Work out the finished part from the listing and answer in its coordinate system (mm). Face numbers are marked on the shaded views. A direction names the side the tool comes from. Round coordinates to 2 decimals unless told otherwise and drop trailing zeros. Order: outer loops, then holes, each group sorted by start corner. A loop starts at its lowest first (then second) coordinate and runs counter-clockwise, first axis right, second up. Notation, with made-up numbers: (-31, -16.75) - (18, -16.75) arc R21 ccw to (18, 5.25) - close; hole circle Ø7 at (86.5, -6.5). An arc over 180 degrees is marked (long way). Answer in a Markdown table with one row per item.
from build123d import *

# Parameters (mm, degrees)
SZKIC1_R                    = 15
DODANIE_WYCI_GNI_CIE1_DEPTH = 53
SFAZOWANIE1_SIZE            = 1
WYTNIJ_WYCI_GNI_CIE1_DEPTH  = 35
SZKIC3_R                    = 30
DODANIE_WYCI_GNI_CIE2_DEPTH = 10
SZKIC4_R                    = 2.5
WYTNIJ_WYCI_GNI_CIE2_DEPTH  = 61.406953242
SZYK_KO_OWY1_COUNT          = 6


with BuildPart() as part:
    # Szkic1 → Dodanie-wyciągnięcie1 (new body)
    with BuildSketch(Plane.XY):
        Circle(SZKIC1_R)
    extrude(amount=DODANIE_WYCI_GNI_CIE1_DEPTH)

    # Sfazowanie1
    sfazowanie1_edges = [part.edges().sort_by_distance(p)[0] for p in [
        (-15, 0, 0),
    ]]
    chamfer(sfazowanie1_edges, length=SFAZOWANIE1_SIZE)

    # Szkic2 → Wytnij-wyciągnięcie1 (cut)
    with BuildSketch(Plane(origin=(0, 0, 4), x_dir=(-1, 0, 0), z_dir=(0, 0, -1))):
        with BuildLine():
            Line((-2.39, 14.808372632), (-2.39, 12.418372632))
            Line((-2.39, 12.418372632), (2.39, 12.418372632))
            Line((2.39, 12.418372632), (2.39, 14.808372632))
            ThreePointArc((2.39, 14.808372632), (0, 15), (-2.39, 14.808372632))
        make_face()
    extrude(amount=-WYTNIJ_WYCI_GNI_CIE1_DEPTH, mode=Mode.SUBTRACT)

    # Szkic3 → Dodanie-wyciągnięcie2 (add)
    with BuildSketch(Plane.XY.offset(53)):
        Circle(SZKIC3_R)
    extrude(amount=-DODANIE_WYCI_GNI_CIE2_DEPTH)

    # Szkic4 → Wytnij-wyciągnięcie2 (cut, through all)
    with BuildSketch(Plane(origin=(0, 0, 43), x_dir=(-1, 0, 0), z_dir=(0, 0, -1))):
        with Locations((-25, 0)):
            Circle(SZKIC4_R)
    wytnij_wyci_gni_cie2 = extrude(amount=-WYTNIJ_WYCI_GNI_CIE2_DEPTH, mode=Mode.SUBTRACT)

    # Szyk kołowy1: Wytnij-wyciągnięcie2 ×6 about axis
    szyk_ko_owy1_axis = Axis((0, 0, 0), (0, 0, 1))
    for i in range(1, SZYK_KO_OWY1_COUNT):
        add(wytnij_wyci_gni_cie2.rotate(szyk_ko_owy1_axis, i * 360 / SZYK_KO_OWY1_COUNT), mode=Mode.SUBTRACT)


solid = part.part
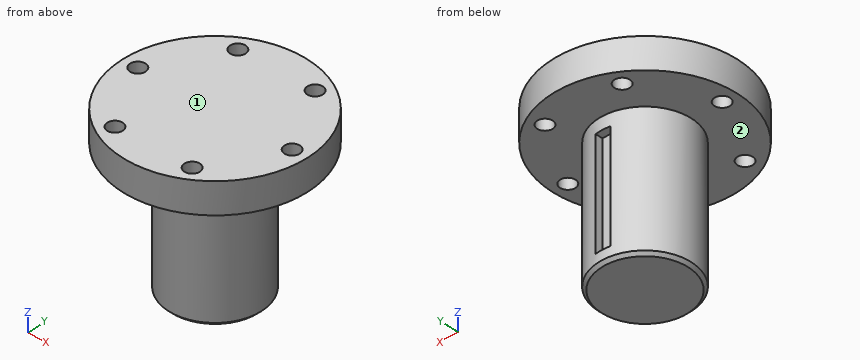
1) Find the intervals of material crossed by probe 1 along Y at (x, z) = (-11, 43.5); probe 2 along Y at (x, z) = (12, 49); probe 3 along Z at (x, y) = (20.5, 8), in increasing order. Write a range as from..to.
Filled in:
| item | result |
|---|---|
| probe 1 | y = -27.91..-23.65, -19.65..19.65, 23.65..27.91 |
| probe 2 | y = -27.5..-24.1, -19.2..19.2, 24.1..27.5 |
| probe 3 | z = 43..53 |
2) Find section B-B, the plane x = 0. Give the vertices of the cut face in (y, z), then the cut area to 3 significant figures.
Filled in:
| item | result |
|---|---|
| outline | (-30, 43) - (-15, 43) - (-15, 1) - (-14, 0) - (14, 0) - (15, 1) - (15, 4) - (12.42, 4) - (12.42, 39) - (15, 39) - (15, 43) - (30, 43) - (30, 53) - (-30, 53) - close |
| area | 1,800 mm^2 |
3) Which of the six approach directions +Z, -Z, +X, -X, +Y, -Y give full straight-line access (tool end or side, diameter ignored) to the marked faces 1 and 2?
Filled in:
| item | result |
|---|---|
| face 1 | +Z, +X, -X, +Y, -Y |
| face 2 | -Z |
4) Find section A-A, the plane y = 0. Give the vertices of the cut face in (x, z), then the cut area to 3 significant figures.
Filled in:
| item | result |
|---|---|
| outline | (-30, 43) - (-27.5, 43) - (-27.5, 53) - (-30, 53) - close; (-22.5, 43) - (-15, 43) - (-15, 1) - (-14, 0) - (14, 0) - (15, 1) - (15, 43) - (22.5, 43) - (22.5, 53) - (-22.5, 53) - close; (27.5, 43) - (30, 43) - (30, 53) - (27.5, 53) - close |
| area | 1,790 mm^2 |
5) Find section C-C, the plane x = -25. Give the vertices of the cut face in (y, z).
Filled in:
| item | result |
|---|---|
| outline | (-16.58, 43) - (-2.5, 43) - (-2.5, 53) - (-16.58, 53) - close; (2.5, 43) - (16.58, 43) - (16.58, 53) - (2.5, 53) - close |
6) Each of these flat-tipped pins is pushed along its axis until it touches: pin 1 (6 mm diameter, centred on x = 14, y = -20, fed in from -Z); pin 2 (1 mm diameter, centred on x = 0, z = 11, fed in from +Y); pin 3 (1.2 mm diameter, centred on y = 13.5, z = 15.5, fed in from +X). Where does it stop, or does it pass through?
Filled in:
| item | result |
|---|---|
| pin 1 | stops at z = 43 |
| pin 2 | stops at y = 12.42 |
| pin 3 | stops at x = 7.65 |
7) Find section D-D, the plane y = 21.5. Give the vertices of the cut face in (x, z), then the cut area to 3 significant figures.
Filled in:
| item | result |
|---|---|
| outline | (-20.92, 43) - (-15, 43) - (-15, 53) - (-20.92, 53) - close; (-10, 43) - (10, 43) - (10, 53) - (-10, 53) - close; (15, 43) - (20.92, 43) - (20.92, 53) - (15, 53) - close |
| area | 319 mm^2 |
